CAD build for the part. Positions are in the model's coordinates, mm. Face numbers are marked on the shaded views. A direction names the side the tool comes from. Give positions to 0.01 mm unless a question says otherwise; leave off trailing zeros. Order: outer loops, then holes, each group sorted by start corner. A loop starts at its lowest first (then second) coordinate and runs counter-clockwise, first axis right, second up. Notation, with made-up numbers: M -29.75,34 L -2.75,34 A10 cw -2.75,46 Z; hole C 51,-28 d9. An arc over 180 degrees is marked long. Put each result on its own line as item: value. Start each with the question number.
1) Two-plate mould, pull along X, no slides. Class the marked faces 3, 4 and 5: released by +X, released by -X, zero draft, split by the parting line, or undercut.
2) Pin check, flat tips, straight feed: pin 1 (1.5 mm diameter, centred on y = 24, z = 12, fed in from -X); pin 2 (1 mm diameter, centred on x = 28, z = 32, fed in from +Y); pin 3 (6 mm diameter, centred on y = 20, z = 15.5, fed in from -X); pin 4 (6 mm diameter, centred on x = -33.5, y = -20, fed in from -Z). Stop position of each tip, or through.
3) Cut at A-A (z = 55.5). Write the cut outline in (x, y), and give its area (3 significant figures).
4) Drill centre lines: line 1 (X direction, y = 5.5, z = 45.5); line 2 (Y direction, x = 23, z = 41); line 3 (Z direction, x = 13, y = 4.5). Where is each one in solid material? Low to high. Write a range as [from, to].
5) Tool access for the marked faces 1 and 2: list every direction of +Z, -Z, +X, -X, +Y, -Y with a clear straight run to the whole face (end or side of a thin tool).
```python
from build123d import *

# Parameters (mm, degrees)
F1_DEPTH = 76.2
F2_T     = -5.08
F3_R     = 5.08


with BuildPart() as f1:
    # F0 (on Top) → F1 (new body)
    with BuildSketch(Plane.XY):
        Polygon((-43.242968, -14.145307), (-15.902303, -42.628169), (23.413121, -39.01115), (45.097987, -6.017939), (32.823149, 31.506902), (-4.168189, 45.306404), (-38.020797, 24.989259), align=None)
    extrude(amount=F1_DEPTH)

    # F2
    f2_openings = [f1.faces().sort_by_distance(p)[0] for p in [
        (0, 0, 76.2),
    ]]
    offset(amount=F2_T, openings=f2_openings)

    # F3
    f3_edges = [f1.edges().sort_by_distance(p)[0] for p in [
        (3.755409, -40.819659, 0),
        (34.255554, -22.514545, 0),
        (38.960568, 12.744482, 0),
        (14.32748, 38.406653, 0),
        (-21.094493, 35.147832, 0),
        (-40.631882, 5.421976, 0),
        (-29.572636, -28.386738, 0),
    ]]
    fillet(f3_edges, radius=F3_R)


solid = f1.part
```
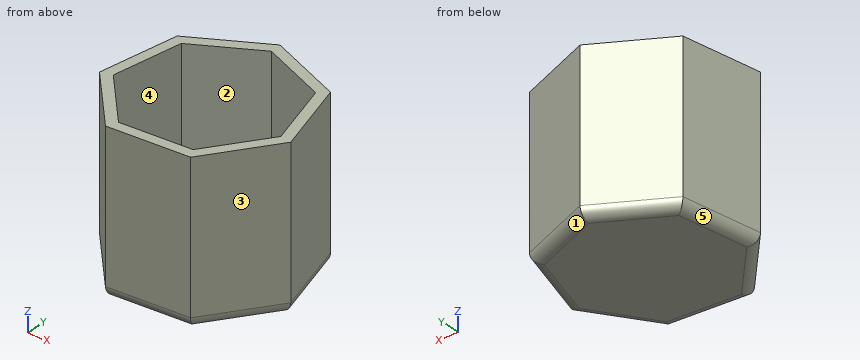
Solution:
1. face 3: released by +X
1. face 4: undercut
1. face 5: released by -X
2. pin 1: x = -38.25
2. pin 2: y = 33.49
2. pin 3: x = -39.09
2. pin 4: z = 0
3. outline: M -43.24,-14.15 L -15.9,-42.63 L 23.41,-39.01 L 45.1,-6.02 L 32.82,31.51 L -4.17,45.31 L -38.02,24.99 Z; hole M -37.88,-12.39 L -13.93,-37.35 L 20.51,-34.18 L 39.51,-5.27 L 28.76,27.6 L -3.65,39.69 L -33.31,21.89 Z
3. area: 1,320 mm²
4. line 1: [-40.62, -35.5], [35.99, 41.33]
4. line 2: [-39.05, -30.39], [29.75, 35.17]
4. line 3: [0, 5.08]
5. face 1: -Z, +X, +Y
5. face 2: +Z
